from build123d import *

# Parameters (mm, degrees)
MODEL_W               = 126
MODEL_H               = 215
MODEL_R               = 4.5
MODEL_R_2             = 6.25
MODEL_R_3             = 5.25
MODEL_R_4             = 2.750009003
MODEL_R_5             = 1.25
MODEL_R_6             = 2.625
MODEL_R_7             = 1.75
TABAN_FLAN_1_DEPTH    = 4
IZIM1_W               = 102.176444729
IZIM1_H               = 22.108353538
SEKME1_DEPTH          = 4
IZIM4_R               = 4.25
KES_EKSTR_ZYON1_DEPTH = 10
KES_EKSTR_ZYON2_DEPTH = 10
KES_EKSTR_ZYON4_DEPTH = 10
RADYUS1_R             = 3


# Sheet-metal steps are written as plain solids
with BuildPart() as part:
    # Model → Taban-Flanş1 (new body)
    with BuildSketch(Plane.XY):
        with Locations((2161.892923165, 1693.121210327)):
            Rectangle(MODEL_W, MODEL_H)
        with Locations((2129.437918581, 1602.511715112)):
            Circle(MODEL_R, mode=Mode.SUBTRACT)
        with Locations((2194.437918581, 1602.511715112)):
            Circle(MODEL_R, mode=Mode.SUBTRACT)
        with Locations((2161.892918569, 1777.197615102)):
            Circle(MODEL_R_2, mode=Mode.SUBTRACT)
        with Locations((2161.892918569, 1648.515095807)):
            Circle(MODEL_R_3, mode=Mode.SUBTRACT)
        with Locations((2197.838423148, 1781.897610313)):
            Circle(MODEL_R_4, mode=Mode.SUBTRACT)
        with Locations((2203.017232274, 1786.156601204)):
            Circle(MODEL_R_5, mode=Mode.SUBTRACT)
        with Locations((2197.833609474, 1774.397615119)):
            Circle(MODEL_R_4, mode=Mode.SUBTRACT)
        with Locations((2203.012418599, 1778.65660601)):
            Circle(MODEL_R_5, mode=Mode.SUBTRACT)
        with Locations((2197.834704915, 1766.897610313)):
            Circle(MODEL_R_4, mode=Mode.SUBTRACT)
        with Locations((2203.013514041, 1771.156601204)):
            Circle(MODEL_R_5, mode=Mode.SUBTRACT)
        with Locations((2197.834104915, 1759.397610313)):
            Circle(MODEL_R_4, mode=Mode.SUBTRACT)
        with Locations((2203.012914041, 1763.656601204)):
            Circle(MODEL_R_5, mode=Mode.SUBTRACT)
        with Locations((2197.835304915, 1751.897610313)):
            Circle(MODEL_R_4, mode=Mode.SUBTRACT)
        with Locations((2203.014114041, 1756.156601204)):
            Circle(MODEL_R_5, mode=Mode.SUBTRACT)
        with Locations((2197.836004915, 1744.397610313)):
            Circle(MODEL_R_4, mode=Mode.SUBTRACT)
        with Locations((2203.014814041, 1748.656601204)):
            Circle(MODEL_R_5, mode=Mode.SUBTRACT)
        with Locations((2197.833623148, 1736.897610313)):
            Circle(MODEL_R_4, mode=Mode.SUBTRACT)
        with Locations((2203.012432274, 1741.156601204)):
            Circle(MODEL_R_5, mode=Mode.SUBTRACT)
        with Locations((2197.833623148, 1729.397610313)):
            Circle(MODEL_R_4, mode=Mode.SUBTRACT)
        with Locations((2203.012432274, 1733.656601204)):
            Circle(MODEL_R_5, mode=Mode.SUBTRACT)
        with Locations((2208.53221406, 1742.933219427)):
            Circle(MODEL_R_6, mode=Mode.SUBTRACT)
        with Locations((2163.619323241, 1734.111700763)):
            Circle(MODEL_R_7, mode=Mode.SUBTRACT)
        with Locations((2120.695323241, 1743.382400763)):
            Circle(MODEL_R_7, mode=Mode.SUBTRACT)
    extrude(amount=-TABAN_FLAN_1_DEPTH)

    # Çizim1 → Sekme1 (add)
    with BuildSketch(Plane.XY):
        with Locations((2155.462798754, 1603.699676968)):
            Rectangle(IZIM1_W, IZIM1_H)
    extrude(amount=-SEKME1_DEPTH)

    # Çizim4 → Kes-Ekstrüzyon1 (cut)
    with BuildSketch(Plane.XY):
        with Locations((2129.392923165, 1601.621210327)):
            Circle(IZIM4_R)
        with Locations((2194.392923165, 1601.621210327)):
            Circle(IZIM4_R)
    extrude(amount=-KES_EKSTR_ZYON1_DEPTH, mode=Mode.SUBTRACT)

    # Çizim7 → Kes-Ekstrüzyon2 (cut)
    with BuildSketch(Plane.XY):
        with BuildLine():
            ThreePointArc((2115.489264274, 1685.628682491), (2107.413399384, 1672.236382403), (2103.111338467, 1657.20090545))
            ThreePointArc((2103.111338467, 1657.20090545), (2109.85599076, 1648.117422338), (2118.939473872, 1654.862074631))
            ThreePointArc((2118.939473872, 1654.862074631), (2122.083117431, 1665.848943761), (2127.984391527, 1675.635094799))
            ThreePointArc((2127.984391527, 1675.635094799), (2126.733621746, 1686.879452271), (2115.489264274, 1685.628682491))
        make_face()
    extrude(amount=-KES_EKSTR_ZYON2_DEPTH, mode=Mode.SUBTRACT)

    # Çizim9 → Kes-Ekstrüzyon4 (cut)
    with BuildSketch(Plane.XY):
        with BuildLine():
            Line((2109.684510436, 1733.919137473), (2109.684510436, 1713.919137473))
            ThreePointArc((2109.684510436, 1713.919137473), (2107.684510436, 1711.919137473), (2105.684510436, 1713.919137473))
            Line((2105.684510436, 1713.919137473), (2105.684510436, 1733.919137473))
            ThreePointArc((2105.684510436, 1733.919137473), (2107.684510436, 1735.919137473), (2109.684510436, 1733.919137473))
        make_face()
        with BuildLine():
            Line((2130.684510436, 1733.919137473), (2130.684510436, 1713.919137473))
            ThreePointArc((2130.684510436, 1713.919137473), (2128.684510436, 1711.919137473), (2126.684510436, 1713.919137473))
            Line((2126.684510436, 1713.919137473), (2126.684510436, 1733.919137473))
            ThreePointArc((2126.684510436, 1733.919137473), (2128.684510436, 1735.919137473), (2130.684510436, 1733.919137473))
        make_face()
    extrude(amount=-KES_EKSTR_ZYON4_DEPTH, mode=Mode.SUBTRACT)

    # Radyus1
    radyus1_edges = [part.edges().sort_by_distance(p)[0] for p in [
        (2098.892923165, 1800.621210327, -2),
        (2224.892923165, 1800.621210327, -2),
    ]]
    fillet(radyus1_edges, radius=RADYUS1_R)


solid = part.part
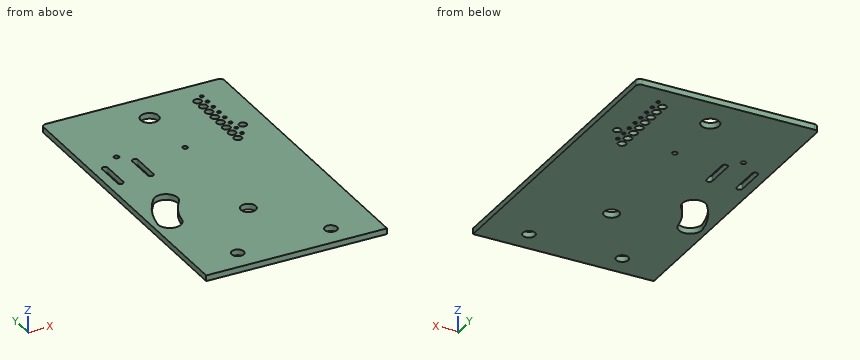
The model under review builds one solid part; all positions refer to its coordinate system, in mm. Give positions to 0.01 mm unless a question says otherwise; leave off trailing zeros. Write each loop counter-clockwise with the first axis right and the second up, starting at its lowest first coordinate (ties: lowest second). Pieces come first, ordered by that corner, then holes.
1. Wall thickness on L1, parallel to Y at x = 2160, z = -2.7; L2, parallel to Y at x = 2166, z = -2.85; L3, parallel to X at y = 1774.5, z = -0.4: over which ranges is each line inside the solid? List them lowest first.
2. Add section A-A, the plane y = 1669. Write out the cut boundary in (x, z), plus the area to 3 significant figures.
3. Add section B-B, the plane z = -1.9. Count the separate pieces of the cut face and the enclosed holes in it, plus the area to 3 significant figures.
Worked answers:
1. L1: y = 1585.62 to 1643.62, 1653.41 to 1771.24, 1783.15 to 1800.62
1. L2: y = 1585.62 to 1645.24, 1651.79 to 1772.49, 1781.91 to 1800.62
1. L3: x = 2098.89 to 2156.26, 2167.53 to 2195.09, 2200.58 to 2224.89
2. outline: (2098.89, -4) - (2106.12, -4) - (2106.12, 0) - (2098.89, 0) - close; (2123.61, -4) - (2224.89, -4) - (2224.89, 0) - (2123.61, 0) - close
2. area: 434 mm2
3. separate pieces: 1
3. enclosed holes: 26
3. area: 25,700 mm2
